For this review, use the dimensioned drawing (mm, ordinates from the lowest corner) and the shaded views. A direction names the side the tool comes from. Round coordinates to 2 decimals unless told otherwise and drop trailing zeros. Loops run counter-clockwise (first coordinate to the right, second up) from the corner with the lowest first, then second, coordinate; pieces in that order, holes last.
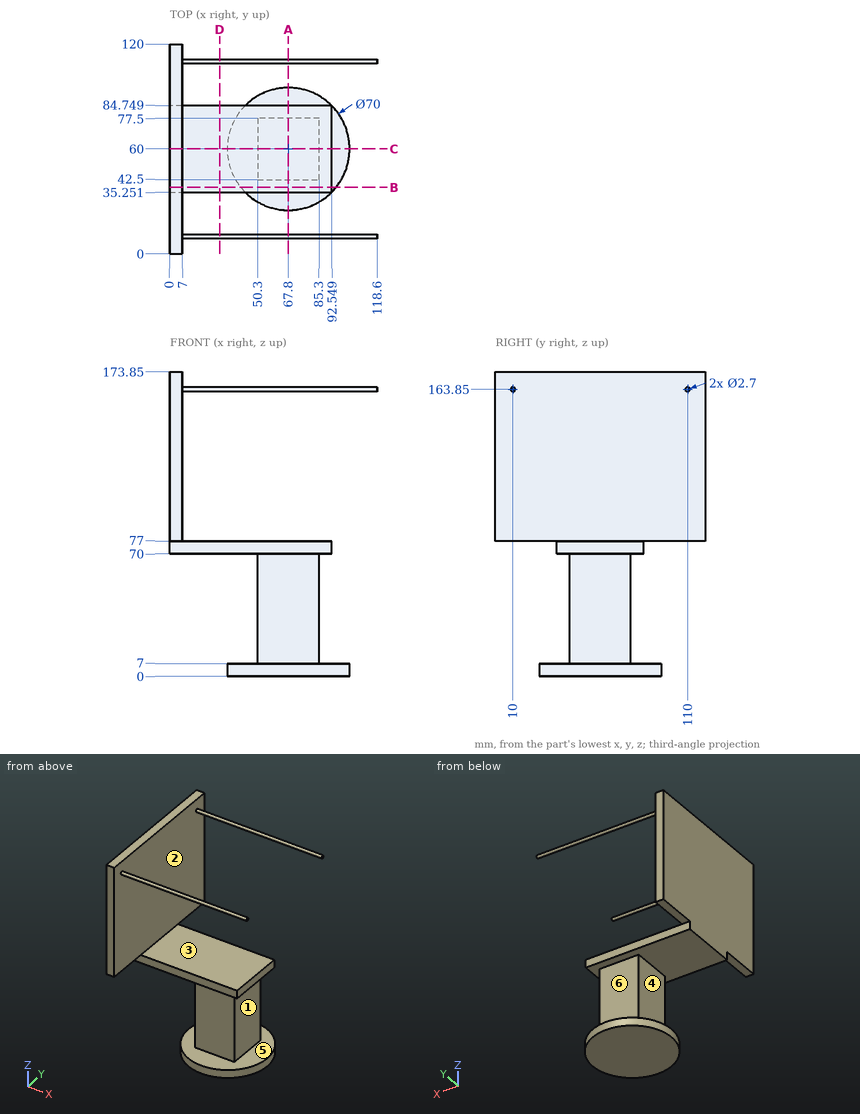
(1) Insertion check: pin 1 Ø21 at (x, y) = (78.5, 67) entering from +Z; pin 2 Ø3.5 at (x, y) = (5, 19.5) entering from -Z; pin 3 Ø4 at (x, z) = (95, 78) entering from +Y; pin 4 Ø17.5 at (x, z) = (60.5, 31.5) entering from -Y. Each pin has a flat end and moves straight along its axis. Give the tip position at first contact, or say it passes through.
(2) Add section A-A (x = 67.8). Give the boundary of the cut face in (y, z), plus the area to 3 significant figures.
(3) Add section C-C (y = 60). Give the boundary of the cut face in (x, z), plus the area to 3 significant figures.
(4) Add section B-B (y = 38). Give the boundary of the cut face in (x, z).
(5) For L1, parallel to Z at x = 44.5, y = 59; L2, parallel to X at y = 63.5, z = 73.5; L3, parallel to Z at x = 58, y = 68.5, list the stretches that pass through material, from the lowest coordinate up.
(6) Add section D-D (x = 28.5). Give the boundary of the cut face in (y, z), plus the area to 3 significant figures.
(7) For the marked faces 4, 5 and 6, list the 3-axis set-ups (+Z, -Z, +X, -X, +Y, -Y) from which the entire face can be reached by the end or side of a thin tool; tool diameter is ignored.
(8) The part is to be moulded in two halves that separate along Z. For the marked faces 1, 2 and 3, say which applies: pulls with the +Z half, pulls with the -Z half, needs draft (parallel to the pull), parting line crosses it, or undercut.
Outcome:
1. pin 1: stops at z = 77
1. pin 2: stops at z = 77
1. pin 3: passes through
1. pin 4: stops at y = 42.5
2. outline: circle Ø2.7 at (10, 163.85); (25, 0) - (95, 0) - (95, 7) - (77.5, 7) - (77.5, 70) - (84.75, 70) - (84.75, 77) - (35.25, 77) - (35.25, 70) - (42.5, 70) - (42.5, 7) - (25, 7) - close; circle Ø2.7 at (110, 163.85)
2. area: 3,050 mm2
3. outline: (0, 70) - (50.3, 70) - (50.3, 7) - (32.8, 7) - (32.8, 0) - (102.8, 0) - (102.8, 7) - (85.3, 7) - (85.3, 70) - (92.55, 70) - (92.55, 77) - (7, 77) - (7, 173.85) - (0, 173.85) - close
3. area: 4,020 mm2
4. outline: (0, 70) - (92.55, 70) - (92.55, 77) - (7, 77) - (7, 173.85) - (0, 173.85) - close; (40.58, 0) - (95.02, 0) - (95.02, 7) - (40.58, 7) - close
5. L1: z = 0 to 7, 70 to 77
5. L2: x = 0 to 92.55
5. L3: z = 0 to 77
6. outline: circle Ø2.7 at (10, 163.85); (35.25, 70) - (84.75, 70) - (84.75, 77) - (35.25, 77) - close; circle Ø2.7 at (110, 163.85)
6. area: 358 mm2
7. face 4: -X, +Y, -Y
7. face 5: none
7. face 6: +X, -X, +Y
8. face 1: undercut
8. face 2: needs draft
8. face 3: pulls with the +Z half
